```python
from build123d import *

# Parameters (mm, degrees)
F0_W     = 12.7
F0_H     = 50.8
F0_H_2   = 12.7
F1_DEPTH = 12.7
F0_R     = 3.175
F2_DEPTH = 2.54
F3_DEPTH = 11.43
F5_DEPTH = 12.7


with BuildPart() as f1:
    # F0 (on Front) → F1 (new body)
    with BuildSketch(Plane.XZ):
        with Locations((-7.0469496608, 2.5596140835)):
            Rectangle(F0_W, F0_H)
        with Locations((-7.0469496608, 34.3096140835)):
            Rectangle(F0_W, F0_H_2)
    extrude(amount=-F1_DEPTH)

    # F0 (on Front) → F2 (join)
    with BuildSketch(Plane.XZ):
        with Locations((-19.7469496608, 2.5596140835)):
            Rectangle(F0_W, F0_H)
        with Locations((-19.7934154421, -15.6117072329)):
            Circle(F0_R, mode=Mode.SUBTRACT)
        with Locations((-20.4100394858, 20.5467736741)):
            Circle(F0_R, mode=Mode.SUBTRACT)
        with Locations((5.6530503392, 2.5596140835)):
            Rectangle(F0_W, F0_H)
        with Locations((5.9255640863, -15.5349638661)):
            Circle(F0_R, mode=Mode.SUBTRACT)
        with Locations((6.4119519666, 20.6297561526)):
            Circle(F0_R, mode=Mode.SUBTRACT)
    extrude(amount=-F2_DEPTH)

    # F0 (on Front) → F3 (join)
    with BuildSketch(Plane.XZ):
        with Locations((-7.0469496608, 47.0096140835)):
            Rectangle(F0_W, F0_H_2)
    extrude(amount=-F3_DEPTH)

    # F4 (on face) → F5 (cut)
    with BuildSketch(Plane(origin=(-13.3969496608, 0, 0), x_dir=(0, -1, 0), z_dir=(-1, 0, 0))):
        Polygon((0, 53.3596140835), (-11.43, 53.3596140835), (-11.43, 41.9296140835), align=None)
    extrude(amount=-F5_DEPTH, mode=Mode.SUBTRACT)


solid = f1.part
```
Work out the finished part from the listing and answer in its coordinate system (mm). A direction names the side the tool comes from. Coordinates: 2 decimals unless noted, no trailing zeros. Order: outer loops, then holes, each group sorted by start corner. A loop starts at its lowest first (then second) coordinate and runs counter-clockwise, first axis right, second up. Notation, with made-up numbers: (38.5, 59.5) - (46.5, 59.5) arc R12 ccw to (46.5, 77.5) - close; hole circle Ø5 at (49.25, 81.25). An arc over 180 degrees is marked (long way). Answer as a JSON object with one key per item and string values.
1. The mould has two halves that part along Z. Classify faces 6 (the face through (12.003, 1, 2)), 7 (the face through (5.237, 1.252, -18.634)), 8 (the face through (-7, 5, -22.84)): +Z half, -Z half, draft (parallel to the pull), parting line (faces both ways), or undercut.
Output values:
{"face 6": "draft", "face 7": "undercut", "face 8": "-Z half"}
2. Find section C-C on x = -8.5. Determine the outline of the cut face in (y, z), plus the area to 3 significant figures.
Output values:
{"outline": "(0, -22.84) - (12.7, -22.84) - (12.7, 40.66) - (11.43, 40.66) - (11.43, 41.93) - (0, 53.36) - close", "area": "886 mm²"}
3. Each of these flat-tipped pins is pushed along its axis until it touches: P1, Ø8.5, axis at x = -19.79, z = -15.61, coming from the -Y side; P2, Ø4, axis at x = 5.5, z = 1, coming from the +Y side; P3, Ø6.5, axis at y = 6.5, z = 3, coming from the +X side; P4, Ø2, axis at x = 3, y = 1.5, coming from the +Z side. Where does it stop, or does it pass through?
Output values:
{"P1": "stops at y = 0", "P2": "stops at y = 2.54", "P3": "stops at x = -0.7", "P4": "stops at z = 27.96"}
4. Find section D-D on y = 6.75. Determine the outline of the cut face in (x, z), plus the area to 3 significant figures.
Output values:
{"outline": "(-13.4, -22.84) - (-0.7, -22.84) - (-0.7, 46.61) - (-13.4, 46.61) - close", "area": "882 mm²"}
5. Consider line 1 (X direction, y = 11.75, z = 0.5); line 2 (Y direction, x = 5, z = 24); line 3 (Z direction, x = 1.5, y = 0.5). Determine where each line is inside the solid, lowest interval first.
Output values:
{"line 1": "x = -13.4 to -0.7", "line 2": "y = 0 to 2.54", "line 3": "z = -22.84 to 27.96"}
6. A tool of negligible diameter and unlimited length cuts with its end or side. For faces 1 (the face through (-20, 1, 27.96)), 2 (the face through (-20, 2.54, 3)), 3 (the face through (-7, 12.7, 9)), 4 (the face through (6, 2.54, 3)), 5 (the face through (6, 1, 27.96)), from which of +Z, -Z, +X, -X, +Y, -Y can it reach the whole face along a straight path? Write none if from no direction.
Output values:
{"face 1": "+Z, -X, +Y, -Y", "face 2": "+Z, -Z, -X, +Y", "face 3": "+Z, -Z, +X, -X, +Y", "face 4": "+Z, -Z, +X, +Y", "face 5": "+Z, +X, +Y, -Y"}
7. Find section A-A on x = 7. Determine the outline of the cut face in (y, z), plus the area to 3 significant figures.
Output values:
{"outline": "(0, -22.84) - (2.54, -22.84) - (2.54, -18.52) - (0, -18.52) - close; (0, -12.55) - (2.54, -12.55) - (2.54, 17.51) - (0, 17.51) - close; (0, 23.75) - (2.54, 23.75) - (2.54, 27.96) - (0, 27.96) - close", "area": "98.0 mm²"}
8. Find section B-B on z = 12.5. Determine the outline of the cut face in (x, y), plus the area to 3 significant figures.
Output values:
{"outline": "(-26.1, 0) - (12, 0) - (12, 2.54) - (-0.7, 2.54) - (-0.7, 12.7) - (-13.4, 12.7) - (-13.4, 2.54) - (-26.1, 2.54) - close", "area": "226 mm²"}
